The model under review builds one solid part; all positions refer to its coordinate system, in mm. Face numbers are marked on the shaded views. A direction names the side the tool comes from. Give positions to 0.01 mm unless a question says otherwise; leave off trailing zeros. Loops run counter-clockwise (first coordinate to the right, second up) from the corner with the lowest first, then second, coordinate; pieces in that order, holes last. Notation, with made-up numbers: M 80,18.5 L 123,18.5 A32 cw 123,45.5 Z; hole C 15.5,11.5 d1. An arc over 180 degrees is marked long. Write item = value, one per line. Start each with the question number.
1. Draft analysis for pull direction X (two halves, no side actions). For the marked faces 1, 2, 3 and 4, state which applies: pulls with the +X half, pulls with the -X half, needs draft (parallel to the pull), parting line crosses it, or undercut.
2. We need section B-B on z = 5.75. Give the boundary of the cut face in (x, y) (3 decimals).
3. Wall thickness on line 1 along Z through (x, y) = (5, 1.5); line 2 along Y through (x, z) = (0.5, -2); line 3 along Y through (x, z) = (-2, 1.75): over which ranges is each line inside the solid? List them lowest first. Write a range as from..to.
4. We need section D-D on z = -0.5. Give the boundary of the cut face in (x, y) (3 decimals), then the cut area to 3 significant figures.
5. We need section A-A on y = -1. Give the boundary of the cut face in (x, z) (3 decimals).
6. We need section C-C on x = 4. Give the boundary of the cut face in (y, z), then the cut area to 3 significant figures.
7. For pin 1 (4 mm diameter, centred on x = 0.5, z = -0.5, fed in from -Y); pin 2 (0.5 mm diameter, centred on x = -7, z = 3.5, fed in from -Y); pin 3 (4.5 mm diameter, centred on y = 1.5, z = 3.5, fed in from +X) (3 decimals), all flat-tipped, find the tip position at first contact; note any pin that passes through.
8. For the marked faces 5, 6 and 7, list the 3-axis set-ups (+Z, -Z, +X, -X, +Y, -Y) from which the entire face can be reached by the end or side of a thin tool; tool diameter is ignored.
from build123d import *

# Parameters (mm, degrees)
SKETCH1_W           = 14.07
SKETCH1_H           = 13.18
BOSS_EXTRUDE1_DEPTH = 5
SKETCH2_W           = 13.41
SKETCH2_H           = 4.94
SKETCH2_H_2         = 5.888730893
CUT_EXTRUDE1_DEPTH  = 9
BOSS_EXTRUDE2_START = 3.3
BOSS_EXTRUDE2_DEPTH = 0.93
BOSS_EXTRUDE3_START = 3.3
SKETCH5_R           = 6.26
BOSS_EXTRUDE3_DEPTH = 5.6
BOSS_EXTRUDE4_START = 3.3
SKETCH7_R           = 3.2
BOSS_EXTRUDE4_DEPTH = 8.1
BOSS_EXTRUDE5_START = 3.3
SKETCH8_R           = 3.165
BOSS_EXTRUDE5_DEPTH = 8.3


with BuildPart() as part:
    # Sketch1 → Boss-Extrude1 (new body, symmetric)
    with BuildSketch(Plane(origin=(0, 0, 0), x_dir=(1, 0, 0), z_dir=(0, 1, 0))):
        Rectangle(SKETCH1_W, SKETCH1_H)
    extrude(amount=BOSS_EXTRUDE1_DEPTH, both=True)

    # Sketch2 → Cut-Extrude1 (cut)
    with BuildSketch(Plane(origin=(0, 5, 0), x_dir=(1, 0, 0), z_dir=(0, 1, 0))):
        with Locations((0, 3.79)):
            Rectangle(SKETCH2_W, SKETCH2_H)
        with Locations((0, -3.315634554)):
            Rectangle(SKETCH2_W, SKETCH2_H_2)
    extrude(amount=-CUT_EXTRUDE1_DEPTH, mode=Mode.SUBTRACT)

    # Sketch3 → Boss-Extrude2 (add)
    with BuildSketch(Plane.XY.offset(BOSS_EXTRUDE2_START)):
        Polygon((7.035, -5), (7.65, -6.03042467), (7.65, -25.63042467), (5.75, -25.63042467), (5.75, -44.53042467), (3.48, -44.53042467), (3.48, -42.43042467), (-2.448967454, -42.43042467), (-3.48, -44.53042467), (-5.75, -44.53042467), (-5.75, -25.63042467), (-7.65, -25.63042467), (-7.65, -6.03042467), (-7.035, -5), align=None)
    extrude(amount=BOSS_EXTRUDE2_DEPTH)

    # Sketch5 → Boss-Extrude3 (add)
    with BuildSketch(Plane.XY.offset(BOSS_EXTRUDE3_START)):
        with Locations((-1.283039212, -11.96715887)):
            Circle(SKETCH5_R)
    extrude(amount=-BOSS_EXTRUDE3_DEPTH)

    # Sketch7 → Boss-Extrude4 (add)
    with BuildSketch(Plane.XY.offset(BOSS_EXTRUDE4_START)):
        with Locations((-1.877046038, -27.386019249)):
            Circle(SKETCH7_R)
    extrude(amount=-BOSS_EXTRUDE4_DEPTH)

    # Sketch8 → Boss-Extrude5 (add)
    with BuildSketch(Plane.XY.offset(BOSS_EXTRUDE5_START)):
        with Locations((-1.952127879, -38.498131793)):
            Circle(SKETCH8_R)
    extrude(amount=-BOSS_EXTRUDE5_DEPTH)


solid = part.part
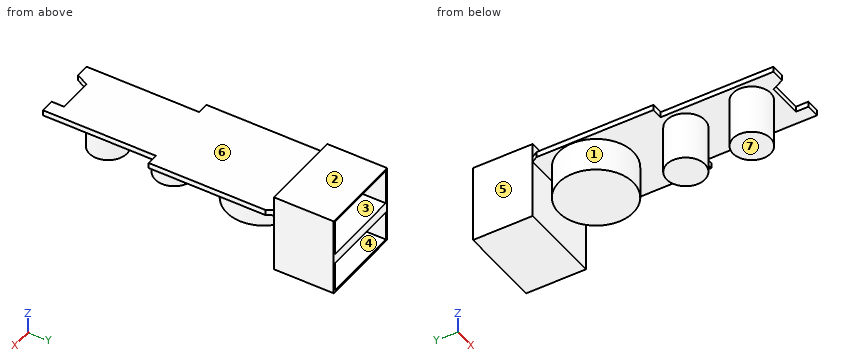
Final values:
q1.face_1 = parting line crosses it
q1.face_2 = needs draft
q1.face_3 = undercut
q1.face_4 = undercut
q2.outline = M -7.035,-5 L 7.035,-5 L 7.035,5 L 6.705,5 L 6.705,-4 L -6.705,-4 L -6.705,5 L -7.035,5 Z
q3.line_1 = -6.59..-6.26, -1.32..0.37, 6.26..6.59
q3.line_2 = -40.5..-36.5, -29.53..-25.24, -17.97..-5.97, -5..-4
q3.line_3 = -41.66..-35.33, -30.58..-24.19, -18.19..-5.75, -5..-4
q4.outline = C -1.283,-11.967 d12.52; M -7.035,-5 L 7.035,-5 L 7.035,5 L -7.035,5 Z; C -1.952,-38.498 d6.33; C -1.877,-27.386 d6.4
q4.area = 327 mm²
q5.outline = M -7.035,-6.59 L 7.035,-6.59 L 7.035,6.59 L -7.035,6.59 Z; hole M -6.705,-6.26 L 6.705,-6.26 L 6.705,-1.32 L -6.705,-1.32 Z; hole M -6.705,0.371 L 6.705,0.371 L 6.705,6.26 L -6.705,6.26 Z
q6.outline = M -44.53,3.3 L -15.33,3.3 L -15.33,-2.3 L -8.61,-2.3 L -8.61,3.3 L -5,3.3 L -5,-6.59 L 5,-6.59 L 5,-6.26 L -4,-6.26 L -4,-1.32 L 5,-1.32 L 5,0.37 L -4,0.37 L -4,6.26 L 5,6.26 L 5,6.59 L -5,6.59 L -5,4.23 L -44.53,4.23 Z
q6.area = 109 mm²
q7.pin_1 = -41.63
q7.pin_2 = -25.63
q7.pin_3 = 7.035
q8.face_5 = +Z, -Z, -X, +Y
q8.face_6 = +Z, +X, -X, -Y
q8.face_7 = -Z, +X, -X, -Y
